from build123d import *

# Parameters (mm, degrees)
F5_DEPTH = 2.54
F6_DEPTH = 2.54


with BuildPart() as f1:
    # F0 (on Front) → F1 (revolve)
    with BuildSketch(Plane.XZ):
        Polygon((0, -15.305464), (0, -7.240309), (-14.847217, -7.240309), (-16.863504, -11.456186), (-18.696494, -11.456186), (-21.079382, -15.305464), align=None)
    revolve(axis=Axis((0, 0, -11.272887), (0, 0, 1)))

    # F2 (on Front) → F3 (revolve)
    with BuildSketch(Plane.XZ):
        Polygon((-4.272232, -7.943824), (0, -7.943824), (0, 25.965976), (-18.298559, 25.965976), (-15.832391, 19.646421), (-11.362462, 9.473482), (-6.892534, 2.383251), (-4.118097, -0.237052), (-4.118097, -3.473896), (-5.813586, -5.169386), (-7.971482, -6.556605), (-7.971482, -7.943824), align=None)
    revolve(axis=Axis((0, 0, 9.011076), (0, 0, -1)))

    # F4 (on Front) → F5 (join)
    with BuildSketch(Plane.XZ):
        Polygon((-16.37111, 13.455632), (-11.964304, 15.659036), (-13.0012, 19.288169), (-19.222574, 16.436707), (-20.389082, 9.437662), (-16.889559, 3.734736), (-12.482752, 2.438617), (-4.576424, 2.438617), (-4.576424, 3.99396), (-7.168663, 5.938139), (-12.223529, 5.938139), (-15.074992, 6.586199), (-16.889559, 9.956109), align=None)
        Polygon((16.889559, 9.956109), (15.074992, 6.586199), (12.223529, 5.938139), (7.168663, 5.938139), (4.576424, 3.99396), (4.576424, 2.438617), (12.482752, 2.438617), (16.889559, 3.734736), (20.389082, 9.437662), (19.222574, 16.436707), (13.0012, 19.288169), (11.964304, 15.659036), (16.37111, 13.455632), align=None)
    extrude(amount=F5_DEPTH)

    # F4 (on Front) → F6 (join)
    with BuildSketch(Plane.XZ):
        Polygon((-16.37111, 13.455632), (-11.964304, 15.659036), (-13.0012, 19.288169), (-19.222574, 16.436707), (-20.389082, 9.437662), (-16.889559, 3.734736), (-12.482752, 2.438617), (-4.576424, 2.438617), (-4.576424, 3.99396), (-7.168663, 5.938139), (-12.223529, 5.938139), (-15.074992, 6.586199), (-16.889559, 9.956109), align=None)
        Polygon((16.889559, 9.956109), (15.074992, 6.586199), (12.223529, 5.938139), (7.168663, 5.938139), (4.576424, 3.99396), (4.576424, 2.438617), (12.482752, 2.438617), (16.889559, 3.734736), (20.389082, 9.437662), (19.222574, 16.436707), (13.0012, 19.288169), (11.964304, 15.659036), (16.37111, 13.455632), align=None)
    extrude(amount=-F6_DEPTH)

    # F7 (on Front) → F8 (revolve, cut)
    with BuildSketch(Plane.XZ):
        Polygon((0, 3.12148), (0, 23.313222), (0, 27.320744), (-15.84477, 27.320744), (-14.53462, 23.236156), (-13.147401, 19.536905), (-8.75454, 9.441033), (-4.614143, 3.12148), align=None)
    revolve(axis=Axis((0, 0, 15.221112), (0, 0, -1)), mode=Mode.SUBTRACT)


solid = f1.part
Source: CAD feature listing. Evaluate the final solid. Frame: model axes, mm. A direction names the side the tool comes from. Coordinates: 2 decimals unless noted, no trailing zeros. Loops run counter-clockwise (first coordinate to the right, second up) from the corner with the lowest first, then second, coordinate; pieces in that order, holes last. Notation, with made-up numbers: (86, -7) - (120, -7) arc R30 cw to (120, 24) - close; hole circle Ø4 at (-24.75, 78). An arc over 180 degrees is marked (long way). Return JSON: item names as keys, results as strings.
Q1. Section A-A, the plane z = 11. Return loops of the section in (x, y), plus the area to 3 significant figures.
Results:
{"outline": "(-20.13, -2.54) - (-16.73, -2.54) - (-16.73, 2.54) - (-20.13, 2.54) - close; circle Ø24.07 at (0, 0); (16.73, -2.54) - (20.13, -2.54) - (20.13, 2.54) - (16.73, 2.54) - close; hole circle Ø18.87 at (0, 0)", "area": "210 mm2"}
Q2. Section B-B, the plane y = 0. Give the number of separate pieces and of enclosed holes in the cut face, plus the area to 3 significant figures.
Results:
{"separate pieces": "1", "enclosed holes": "2", "area": "673 mm2"}
Q3. Mould query, pull axis X, two halves, no side actions, for faces 1 (the flat face through (-17, -2.54, 9)), 2 (the flat face through (14.66, 0.04, 3.08)), 3 (the flat face through (-15.97, -0.04, 8.25)). Classes: released by +X, released by -X, zero draft, split by the parting line, or undercut.
Results:
{"face 1": "zero draft", "face 2": "released by +X", "face 3": "undercut"}
Q4. Section C-C, the plane z = -2. Return loops of the section in (x, y).
Results:
{"outline": "circle Ø8.24 at (0, 0)"}
Q5. Access query for faces 4 (the conical face through (-5.674, 1.787, -5.256)), 5 (the flat face through (-18.664, -0.036, 6.626)), 6 (the flat face through (-10, -12, 25.966)), 7 (the flat face through (-17, 2.54, 9)), 8 (the flat face through (-13.629, -0.036, 6.258)). Directions: +Z, -Z, +X, -X, +Y, -Y. A direction counts if a zero-diameter tool reaches every point of the face in a straight line with its end or side. Return the directions, or none.
Results:
{"face 4": "none", "face 5": "-X, +Y, -Y", "face 6": "+Z, +X, -X, +Y, -Y", "face 7": "-X, +Y", "face 8": "+Y, -Y"}
Q6. Material intervals for line 1 along Y through (x, z) = (-18, 10); line 2 along X through (y, z) = (-2, 8.5); line 3 along Z through (x, y) = (15, 10), sorted ascending.
Results:
{"line 1": "-2.54 to 2.54", "line 2": "-19.81 to -16.11, -10.56 to -7.89, 7.89 to 10.56, 16.11 to 19.81", "line 3": "-15.31 to -11.46, 25.27 to 25.97"}
Q7. Contact query for flat-ended pins moving along their axis: P1, Ø12, axis at y = 0, z = -9, coming from the -X side; P2, Ø4.5, axis at x = 2, y = -0.5, coming from the +Z side; P3, Ø4, axis at y = 2, z = -5.5, coming from the +X side; P4, Ø1.5, axis at x = 13, y = 7, coming from the +Z side. Output: stop coordinate, or through.
Results:
{"P1": "x = -20.89", "P2": "z = 3.12", "P3": "x = 14.87", "P4": "z = 25.97"}
